Work out the finished part from the listing and answer in its coordinate system (mm). A direction names the side the tool comes from. Coordinates: 2 decimals unless noted, no trailing zeros. Order: outer loops, then holes, each group sorted by start corner. A loop starts at its lowest first (then second) coordinate and runs counter-clockwise, first axis right, second up.
1. Flat-ended cylindrical pins translate along their axes: pin 1 Ø1.5 at (x, z) = (2.5, 2) entering from +Y; pin 2 Ø2 at (x, y) = (44, -6.5) entering from -Z; pin 3 Ø1.5 at (y, z) = (10.5, 3) entering from -X. Find the tip coordinate at first contact, or state that the pin passes through.
2. The part is cut by section A-A, the plane z = 2.45. Give the vertices of the cut face in (x, y).
3. Determine the mould class of faces 1 (the cylindrical face through (12, -16, 2)), 2 (the flat face through (59, 10, 2)), 3 (the cylindrical face through (0.253, 7.496, 1.972)) for opening direction X: +X half, -X half, draft (parallel to the pull), parting line (faces both ways), or undercut.
4. The part is cut by section D-D, the plane y = 15.5. Give the vertices of the cut face in (x, z).
5. A tool of negligible diameter and unlimited length cuts with its end or side. For faces 4 (the flat face through (58, -10, 2)), 5 (the cylindrical face through (103.695, -1.532, 1.972)), 6 (the flat face through (5, -13, 2)), from which of +Z, -Z, +X, -X, +Y, -Y can it reach the whole face along a straight path? Write none if from no direction.
6. The part is cut by section B-B, the plane y = -15. Give the vertices of the cut face in (x, z).
7. Find the intervals of material crossed by probe 1 along Y at (x, z) = (100, 1.7); probe 2 along X at (y, z) = (2, 3.8); probe 3 along Y at (x, z) = (0, 2.5), in increasing order.
8. The part is cut by section C-C, the plane x = 0. Give the vertices of the cut face in (y, z), then the cut area to 3 significant figures.
```python
from build123d import *

# Parameters (mm, degrees)
BOSS_EXTRUDE1_DEPTH = 4
SKETCH2_R           = 4
CUT_EXTRUDE1_DEPTH  = 4
SKETCH3_R           = 7.5
CUT_EXTRUDE2_DEPTH  = 4
SKETCH4_W           = 10
SKETCH4_H           = 21.533858591
CUT_EXTRUDE3_DEPTH  = 4


with BuildPart() as part:
    # Sketch1 → Boss-Extrude1 (new body)
    with BuildSketch(Plane.XY):
        with BuildLine():
            ThreePointArc((110, 0), (107.071067812, 7.071067812), (100, 10))
            Line((100, 10), (100, 0))
            Line((100, 0), (100, -10))
            ThreePointArc((100, -10), (107.071067812, -7.071067812), (110, 0))
        make_face()
        with BuildLine():
            Line((100, 0), (100, 10))
            ThreePointArc((100, 10), (90, 0), (100, -10))
            Line((100, -10), (100, 0))
        make_face()
        with BuildLine():
            Line((100, 10), (17.320508076, 10))
            ThreePointArc((17.320508076, 10), (19.318516526, 5.176380902), (20, 0))
            ThreePointArc((20, 0), (19.318516526, -5.176380902), (17.320508076, -10))
            Line((17.320508076, -10), (100, -10))
            ThreePointArc((100, -10), (90, 0), (100, 10))
        make_face()
        with BuildLine():
            Line((0, -10), (0, 0))
            Line((0, 0), (0, 10))
            Line((0, 10), (17.320508076, 10))
            ThreePointArc((17.320508076, 10), (-20, 0), (17.320508076, -10))
            Line((17.320508076, -10), (0, -10))
        make_face()
        with BuildLine():
            Line((0, 10), (0, 0))
            Line((0, 0), (0, -10))
            Line((0, -10), (17.320508076, -10))
            ThreePointArc((17.320508076, -10), (19.318516526, -5.176380902), (20, 0))
            ThreePointArc((20, 0), (19.318516526, 5.176380902), (17.320508076, 10))
            Line((17.320508076, 10), (0, 10))
        make_face()
    extrude(amount=BOSS_EXTRUDE1_DEPTH)

    # Sketch2 → Cut-Extrude1 (cut)
    with BuildSketch(Plane.XY):
        with Locations((100, 0)):
            Circle(SKETCH2_R)
    extrude(amount=CUT_EXTRUDE1_DEPTH, mode=Mode.SUBTRACT)

    # Sketch3 → Cut-Extrude2 (cut)
    with BuildSketch(Plane.XY):
        Circle(SKETCH3_R)
    extrude(amount=CUT_EXTRUDE2_DEPTH, mode=Mode.SUBTRACT)

    # Sketch4 → Cut-Extrude3 (cut)
    with BuildSketch(Plane.XY):
        with Locations((0, -14.149166362)):
            Rectangle(SKETCH4_W, SKETCH4_H)
    extrude(amount=CUT_EXTRUDE3_DEPTH, mode=Mode.SUBTRACT)


solid = part.part
```
Geometry says:
1. pin 1: stops at y = 19.92
1. pin 2: stops at z = 0
1. pin 3: stops at x = -17.46
2. outline: (-5, -19.36) - (-5, -5.59) arc R7.5 cw (long way) to (5, -5.59) - (5, -19.36) arc R20 ccw to (17.32, -10) - (100, -10) arc R10 ccw to (100, 10) - (17.32, 10) arc R20 ccw (long way) to start; hole circle Ø8 at (100, 0)
3. face 1: +X half
3. face 2: draft
3. face 3: undercut
4. outline: (-12.64, 0) - (12.64, 0) - (12.64, 4) - (-12.64, 4) - close
5. face 4: +Z, -Z, +X, -Y
5. face 5: +Z, -Z
5. face 6: +Z, -Z, -Y
6. outline: (-13.23, 0) - (-5, 0) - (-5, 4) - (-13.23, 4) - close; (5, 0) - (13.23, 0) - (13.23, 4) - (5, 4) - close
7. probe 1: y = -10 to -4, 4 to 10
7. probe 2: x = -19.9 to -7.23, 7.23 to 96.54, 103.46 to 109.8
7. probe 3: y = 7.5 to 20
8. outline: (7.5, 0) - (20, 0) - (20, 4) - (7.5, 4) - close
8. area: 50.0 mm2
